Could you check a few things on this model? Use its own coordinates, in mm. Face numbers are marked on the shaded views. A direction names the side the tool comes from. Coordinates: 2 decimals unless noted, no trailing zeros. Loops run counter-clockwise (first coordinate to the right, second up) from the corner with the lowest first, then second, coordinate; pieces in that order, holes last.
from build123d import *

# Parameters (mm, degrees)
HEX_2_DEPTH = 4.0386


with BuildPart() as part:
    # BodySke → BaseBody (revolve)
    with BuildSketch(Plane.XY, mode=Mode.PRIVATE) as basebody_sk:
        Polygon((0, 0), (0, 9.9187), (0.127, 9.9187), (6.058529581, 4.7625), (18.10385, 4.7625), (19.05, 3.81635), (19.05, 0), align=None)
    revolve(basebody_sk.sketch.rotate(Axis((0, 0, 0), (1, 0, 0)), 90), axis=Axis((0, 0, 0), (1, 0, 0)))

    # Sketch2 → PreBroach (revolve, cut)
    with BuildSketch(Plane.XY, mode=Mode.PRIVATE) as prebroach_sk:
        Polygon((0, 2.77876), (4.0386, 2.77876), (5.642917834, 0), (0, 0), align=None)
    revolve(prebroach_sk.sketch.rotate(Axis((0, 0, 0), (1, 0, 0)), 90), axis=Axis((0, 0, 0), (1, 0, 0)), mode=Mode.SUBTRACT)

    # Sketch3 → Hex 2 (cut)
    with BuildSketch(Plane.ZY):
        Polygon((-2.77876, -1.604317834), (-2.77876, 1.604317834), (0, 3.208635668), (2.77876, 1.604317834), (2.77876, -1.604317834), (0, -3.208635668), align=None)
    extrude(amount=-HEX_2_DEPTH, mode=Mode.SUBTRACT)


solid = part.part
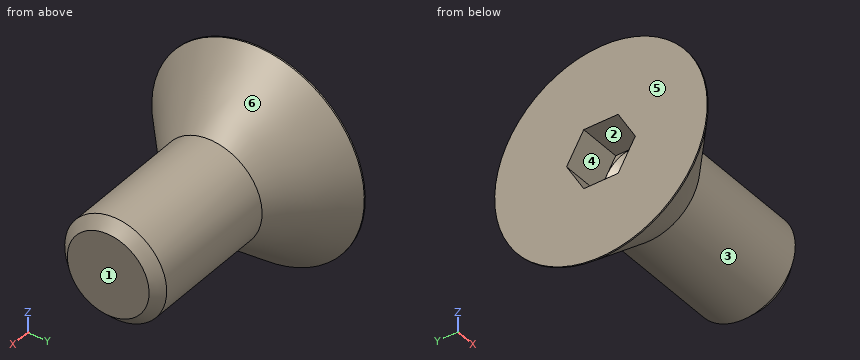
(1) Which directions (+Z, -Z, +X, -X, +Y, -Y) give clear straight access to the entire face, cutting with the end or side of a thin tool? Please do the marked faces 1, 2 and 3.
Answers:
face 1: +Z, -Z, +X, +Y, -Y
face 2: -X
face 3: +X
(2) We'd pull the mould along Y, two halves only. Please class the marked faces 4, 5 and 6: +Y half, -Y half, draft (parallel to the pull), parting line (faces both ways), or undercut.
Answers:
face 4: undercut
face 5: draft
face 6: parting line
(3) For pin 1 (1.6 mm diameter, centred on x = 2.5, y = -0.5, fed in from -Z); pin 2 (0.7 mm diameter, centred on y = -1.5, z = 2, fed in from -X); pin 3 (0.7 mm diameter, centred on y = -1, z = -2, fed in from -X); pin 4 (4 mm diameter, centred on y = -3, z = 4.5, fed in from -X), each with a flat end and sliding along its axis, tell me the tip position at first contact or that it passes through.
Answers:
pin 1: stops at z = -8.54
pin 2: stops at x = 4.04
pin 3: stops at x = 4.15
pin 4: stops at x = 0
(4) I need wall thicknesses on probe 1 along Z at (x, y) = (1.5, 1); probe 2 along X at (y, z) = (-2.5, 8.75); probe 3 along Z at (x, y) = (4.25, -4.25). Which ranges of each line are inside material? Lowest first, please.
Answers:
probe 1: z = -8.67 to -2.78, 2.78 to 8.67
probe 2: x = 0 to 1.07
probe 3: z = -4.7 to 4.7
(5) Imagine slicing it at A-A, the plane x = 8.25. Write out the boundary of the cut face in (y, z) (1 decimal), and give its area (3 significant figures).
Answers:
outline: circle Ø9.5 at (0, 0)
area: 71.3 mm2
